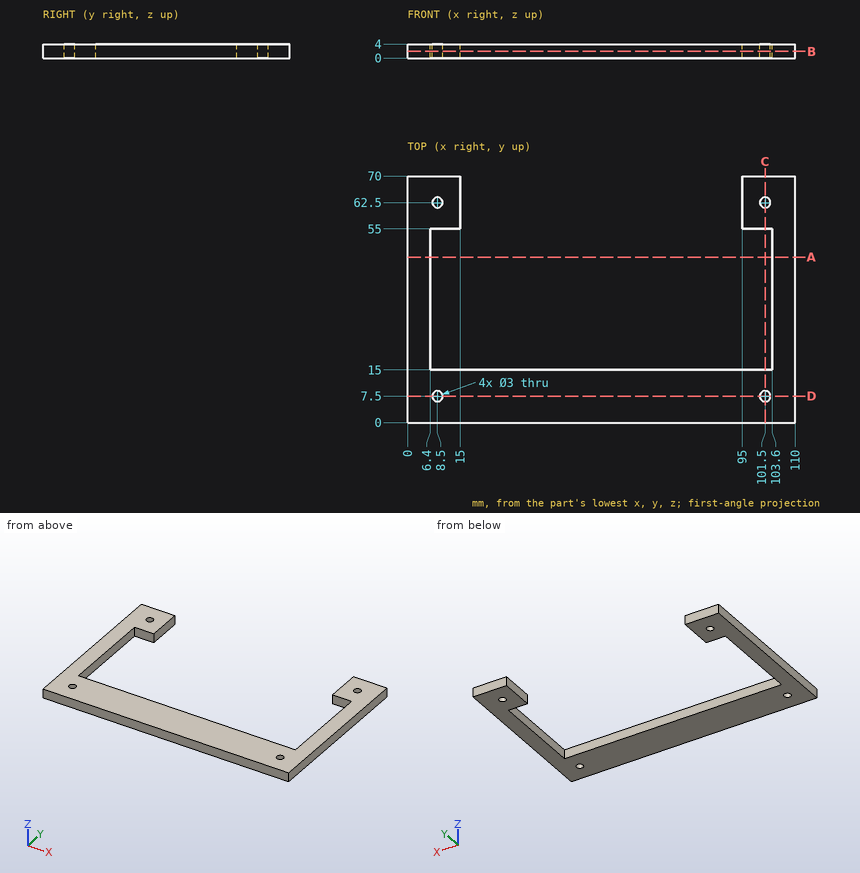
Geometry check sheet. Reference: drawing and pictorial views, mm from the part's lowest x, y, z. Give positions to 0.01 mm unless a question says otherwise; leave off trailing zeros. Order: outer loops, then holes, each group sorted by start corner. A loop starts at its lowest first (then second) coordinate and runs counter-clockwise, first axis right, second up. Notation, with made-up numbers: (-2.5, 20.5) - (50.5, 20.5) arc R16 cw to (50.5, 40.5) - close; hole circle Ø4 at (56.25, -25.5). An arc over 180 degrees is marked (long way). Use one line per item in the form item = value.
1) Sectioned sample at C-C (x = 101.5). Record the boundary of the cut face in (y, z).
Working result:
outline = (0, 0) - (6, 0) - (6, 4) - (0, 4) - close; (9, 0) - (15, 0) - (15, 4) - (9, 4) - close; (55, 0) - (61, 0) - (61, 4) - (55, 4) - close; (64, 0) - (70, 0) - (70, 4) - (64, 4) - close
2) Sectioned sample at A-A (y = 47). Record the boundary of the cut face in (x, z).
Working result:
outline = (0, 0) - (6.4, 0) - (6.4, 4) - (0, 4) - close; (103.6, 0) - (110, 0) - (110, 4) - (103.6, 4) - close
3) Sectioned sample at D-D (y = 7.5). Record the boundary of the cut face in (x, z), and give its area (3 significant figures).
Working result:
outline = (0, 0) - (7, 0) - (7, 4) - (0, 4) - close; (10, 0) - (100, 0) - (100, 4) - (10, 4) - close; (103, 0) - (110, 0) - (110, 4) - (103, 4) - close
area = 416 mm^2
4) Sectioned sample at B-B (z = 1.9). Record the boundary of the cut face in (x, y).
Working result:
outline = (0, 0) - (110, 0) - (110, 70) - (95, 70) - (95, 55) - (103.6, 55) - (103.6, 15) - (6.4, 15) - (6.4, 55) - (15, 55) - (15, 70) - (0, 70) - close; hole circle Ø3 at (8.5, 7.5); hole circle Ø3 at (8.5, 62.5); hole circle Ø3 at (101.5, 7.5); hole circle Ø3 at (101.5, 62.5)
5) Material ranges on probe 1 along Y at (x, z) = (8.5, 3.15); probe 2 along X at (y, z) = (45, 2.8); probe 3 along Y at (x, z) = (8, 3.5), recorded low to high. Write a range as from..to.
Working result:
probe_1 = 0..6, 9..15, 55..61, 64..70
probe_2 = 0..6.4, 103.6..110
probe_3 = 0..6.09, 8.91..15, 55..61.09, 63.91..70
6) Depth check by flat-ended pin: pin 1 Ø2 at (x, z) = (41.5, 1.5) entering from +Y; pin 2 Ø1.2 at (y, z) = (61.5, 1.5) entering from -X; pin 3 Ø2.5 at (x, y) = (8.5, 62.5) entering from +Z. Enter the tip coordinate at first touch or a pass-through.
Working result:
pin_1 = 15
pin_2 = 0
pin_3 = through
